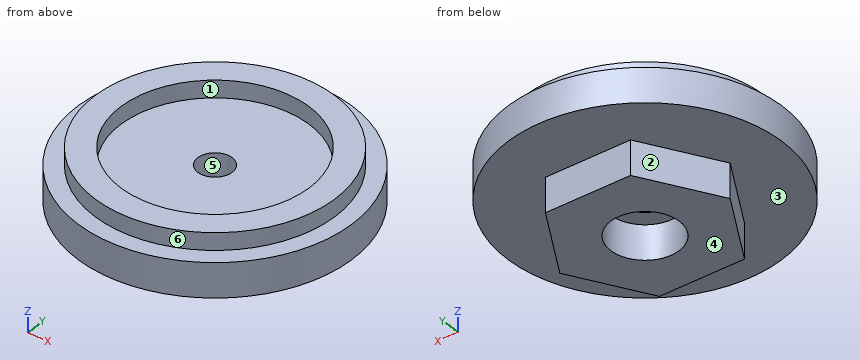
Autodesk Inventor part; units mm, degrees
ref_plane "YZ Plane" through (0, 0, 0) normal (1, 0, 0) x (0, 1, 0)
ref_plane "XZ Plane" through (0, 0, 0) normal (0, 1, 0) x (-1, 0, 0)
ref_plane "XY Plane" through (0, 0, 0) normal (0, 0, 1) x (1, 0, 0)
sketch "Sketch1" plane through (0, 0, 0) normal (0, 0, 1) x (1, 0, 0)
  circle A0 centre (0, 0) radius 25.4
  dimension "d0" = 50.8
extrude "Extrusion1" add sketch "Sketch1" along normal blind 6.35
sketch "Sketch2" plane through (0, 0, 6.35) normal (0, 0, 1) x (1, 0, 0)
  circle A0 centre (0, 0) radius 17.4625
  circle A1 centre (0, 0) radius 22.225
  dimension "d3" = 34.925
  dimension "d4" = 44.45
extrude "Extrusion2" add sketch "Sketch2" along normal blind 3.175
sketch "Sketch3" plane through (0, 0, 0) normal (0, 0, -1) x (-1, 0, 0)
  line L0 (-15.875, 0) -> (-7.9375, 13.7482)
  line L1 (-7.9375, 13.7482) -> (7.9375, 13.7482)
  line L2 (7.9375, 13.7482) -> (15.875, 0)
  line L3 (15.875, 0) -> (7.9375, -13.7482)
  line L4 (7.9375, -13.7482) -> (-7.9375, -13.7482)
  line L5 (-7.9375, -13.7482) -> (-15.875, 0)
  circle A0 centre (0, 0) radius 6.35
  line L6 (0, -35.56) -> (0, 35.56)
  line L7 (-35.56, 0) -> (35.56, 0)
  dimension "d7" = 15.875
  dimension "d8" = 12.7
extrude "Extrusion3" add sketch "Sketch3" along normal blind 6.35 contours L7 A0 L6 L4 L5 | L0 L1 L6 A0 L7 | L1 L2 L7 A0 L6 | L6 A0 L7 L3 L4
hole "Hole1" at (0, 0, 6.35) direction (0, 0, -1) diameter 6.35 end through all
properties part number "2sides"
Source: CAD feature listing. Evaluate the final solid. Frame: model axes, mm. Face numbers are marked on the shaded views. A direction names the side the tool comes from. Give positions to 0.01 mm unless a question says otherwise; leave off trailing zeros. Write each loop counter-clockwise with the first axis right and the second up, starting at its lowest first coordinate (ties: lowest second). Pieces come first, ordered by that corner, then holes. Notation, with made-up numbers: (48.5, 32) - (76.5, 32) arc R27 ccw to (76.5, 56) - close; hole circle Ø10 at (48, 0.25). An arc over 180 degrees is marked (long way). Write item = value, one per line. Start each with the question number.
Q1. Cut plane C-C, the plane y = -20. Return loops of the section in (x, z) (3 decimals).
Q2. Cut plane D-D, the plane x = -12. Return loops of the section in (y, z) (3 decimals).
Q3. Material intervals for probe 1 along X at (y, z) = (0, -2.5) (3 decimals); probe 2 along Y at (x, z) = (0, 4) (3 decimals); probe 3 along Y at (x, z) = (0, 7.3) (1 decimal), sorted ascending.
Q4. Pin query (flat end, axial travel): pin 1 Ø4 at (x, z) = (5, 7.5) entering from +Y; pin 2 Ø3 at (x, z) = (1, -2.5) entering from -Y; pin 3 Ø2 at (x, y) = (5, 1.5) entering from +Z; pin 4 Ø4 at (y, z) = (-19.5, -2.5) entering from -X. Return the tip coordinate at first contact, or that it passes through.
Q5. Draft query along Y for the marked faces 4, 5 and 6. Return one class per face: +Y half, -Y half, draft (parallel to the pull), parting line (faces both ways), or undercut.
Q6. Reachability of the marked faces 1, 2 and 3 from +Z, -Z, +X, -X, +Y, -Y: full face, straight path, thin tool, end or side. Return the list, or none.
Computed values:
q1.outline = (-15.658, 0) - (15.658, 0) - (15.658, 6.35) - (9.693, 6.35) - (9.693, 9.525) - (-9.693, 9.525) - (-9.693, 6.35) - (-15.658, 6.35) - close
q2.outline = (-22.387, 0) - (-6.712, 0) - (-6.712, -6.35) - (6.712, -6.35) - (6.712, 0) - (22.387, 0) - (22.387, 6.35) - (18.707, 6.35) - (18.707, 9.525) - (12.686, 9.525) - (12.686, 6.35) - (-12.686, 6.35) - (-12.686, 9.525) - (-18.707, 9.525) - (-18.707, 6.35) - (-22.387, 6.35) - close
q3.probe_1 = -15.875 to -6.35, 6.35 to 15.875
q3.probe_2 = -25.4 to -3.175, 3.175 to 25.4
q3.probe_3 = -22.2 to -17.5, 17.5 to 22.2
q4.pin_1 = 25.18
q4.pin_2 = -13.75
q4.pin_3 = 6.35
q4.pin_4 = through
q5.face_4 = draft
q5.face_5 = undercut
q5.face_6 = parting line
q6.face_1 = +Z
q6.face_2 = -Z, -X, +Y
q6.face_3 = -Z
